```python
from build123d import *

# Parameters (mm, degrees)
SKETCH1_W           = 40
SKETCH1_H           = 10
BOSS_EXTRUDE1_DEPTH = 312.997959
SKETCH2_W           = 230.9
SKETCH2_H           = 1.2
CUT_EXTRUDE1_DEPTH  = 316.701951749
SKETCH3_R           = 1.9177
CUT_EXTRUDE2_DEPTH  = 316.701951749
CUT_EXTRUDE3_DEPTH  = 4.3
SKETCH5_R           = 2.762258299
CUT_EXTRUDE4_DEPTH  = 316.701951749
SKETCH6_W           = 3.15468
SKETCH6_H           = 6.8326
CUT_EXTRUDE5_DEPTH  = 15


with BuildPart() as part:
    # Sketch1 → Boss-Extrude1 (new body)
    with BuildSketch(Plane(origin=(0, 0, 0), x_dir=(0, 0, -1), z_dir=(1, 0, 0))):
        with Locations((20, 5)):
            Rectangle(SKETCH1_W, SKETCH1_H)
    extrude(amount=BOSS_EXTRUDE1_DEPTH)

    # Sketch2 → Cut-Extrude1 (cut, through all)
    with BuildSketch(Plane(origin=(0, 0, -40), x_dir=(-1, 0, 0), z_dir=(0, 0, -1))):
        with Locations((-156.4989795, 2.6)):
            Rectangle(SKETCH2_W, SKETCH2_H)
    extrude(amount=-CUT_EXTRUDE1_DEPTH, mode=Mode.SUBTRACT)

    # Sketch3 → Cut-Extrude2 (cut, through all)
    with BuildSketch(Plane(origin=(0, 10, 0), x_dir=(1, 0, 0), z_dir=(0, 1, 0))):
        with Locations(Location((294.997959, 25.5, 0), (0, 0, 270))):
            Circle(SKETCH3_R)
        with Locations(Location((294.997959, 14.5, 0), (0, 0, 270))):
            Circle(SKETCH3_R)
        with Locations(Location((18, 14.5, 0), (0, 0, 90))):
            Circle(SKETCH3_R)
        with Locations(Location((18, 25.5, 0), (0, 0, 90))):
            Circle(SKETCH3_R)
    extrude(amount=-CUT_EXTRUDE2_DEPTH, mode=Mode.SUBTRACT)

    # Sketch4 → Cut-Extrude3 (cut)
    with BuildSketch(Plane.XZ):
        Polygon((14.5837, -12.527598275), (14.5837, -16.472401725), (18, -18.444803449), (21.4163, -16.472401725), (21.4163, -12.527598275), (18, -10.555196551), align=None)
        Polygon((14.5837, -23.527598275), (14.5837, -27.472401725), (18, -29.444803449), (21.4163, -27.472401725), (21.4163, -23.527598275), (18, -21.555196551), align=None)
        Polygon((298.414259, -12.527598275), (294.997959, -10.555196551), (291.581659, -12.527598275), (291.581659, -16.472401725), (294.997959, -18.444803449), (298.414259, -16.472401725), align=None)
        Polygon((291.581659, -23.527598275), (291.581659, -27.472401725), (294.997959, -29.444803449), (298.414259, -27.472401725), (298.414259, -23.527598275), (294.997959, -21.555196551), align=None)
    extrude(amount=-CUT_EXTRUDE3_DEPTH, mode=Mode.SUBTRACT)

    # Sketch5 → Cut-Extrude4 (cut, through all)
    with BuildSketch(Plane.XY):
        with Locations((7, 5)):
            Circle(SKETCH5_R)
        with Locations(Location((305.997959, 5, 0), (0, 0, 180))):
            Circle(SKETCH5_R)
    extrude(amount=-CUT_EXTRUDE4_DEPTH, mode=Mode.SUBTRACT)

    # Sketch6 → Cut-Extrude5 (cut)
    with BuildSketch(Plane.ZY):
        with Locations((-31.42266, 5)):
            Rectangle(SKETCH6_W, SKETCH6_H)
        with Locations((-8.57734, 5)):
            Rectangle(SKETCH6_W, SKETCH6_H)
    extrude(amount=-CUT_EXTRUDE5_DEPTH, mode=Mode.SUBTRACT)


solid = part.part
```
Can you work these out from the model? Positions are in its coordinate system, mm. A direction names the side the tool comes from. Coordinates: 2 decimals unless noted, no trailing zeros. Loops run counter-clockwise (first coordinate to the right, second up) from the corner with the lowest first, then second, coordinate; pieces in that order, holes last. Notation, with made-up numbers: (51.25, 79) -> (78.25, 79) arc R22 cw to (78.25, 105) -> close; hole circle Ø8 at (-31, 38.5). An arc over 180 degrees is marked (long way). Put each result on its own line as item: value. Start each with the question number.
Q1. I want a section at B-B (z = -3). Write out the boundary of the cut face in (x, y).
Q2. I want a section at C-C (x = 95.5). Write out the boundary of the cut face in (y, z).
Q3. I want a section at A-A (x = 7). Write out the boundary of the cut face in (y, z).
Q4. I'm going to push a flat-ended pin straight in: P1, Ø2, axis at x = 293.5, z = -15.5, coming from the -Y side. Where does the tip first touch, or does it pass through?
Q5. For faces 4 (the face through (296.5, 4.3, -16.2)), 5 (the face through (9.1, 7.2, -29.845)), 6 (the face through (158, 2, -20)), 7 (the face through (154, 5, -40)), which set-ups out of +Z, -Z, +X, -X, +Y, -Y let a thin tool reach every point of the face, with its end or its side?
Q6. If I drill on line 1 (X direction, y = 8.4, z = -14.5); line 2 (X direction, y = 0.5, z = -25); line 3 (Y direction, x = 236, z = -22.5), over which ranges is the centre line in solid material (lowest first)? Write a range as [from, to].
Q7. Thinking about a two-plate mould opening in Y: for faces 1 (the face through (154, 10, -20)), 2 (the face through (9.1, 7.2, -7)), 3 (the face through (154, 5, 0)), which applies, pulls with the +Y half, pulls with the -Y half, needs draft (parallel to the pull), parting line crosses it, or undercut?
Taken from the geometry:
1. outline: (0, 0) -> (313, 0) -> (313, 10) -> (0, 10) -> close; hole circle Ø5.52 at (7, 5); hole (41.05, 2) -> (271.95, 2) -> (271.95, 3.2) -> (41.05, 3.2) -> close; hole circle Ø5.52 at (306, 5)
2. outline: (0, -40) -> (2, -40) -> (2, 0) -> (0, 0) -> close; (3.2, -40) -> (10, -40) -> (10, 0) -> (3.2, 0) -> close
3. outline: (0, -40) -> (2.24, -40) -> (2.24, -33) -> (1.58, -33) -> (1.58, -29.85) -> (2.24, -29.85) -> (2.24, -10.15) -> (1.58, -10.15) -> (1.58, -7) -> (2.24, -7) -> (2.24, 0) -> (0, 0) -> close; (7.76, -40) -> (10, -40) -> (10, 0) -> (7.76, 0) -> (7.76, -7) -> (8.42, -7) -> (8.42, -10.15) -> (7.76, -10.15) -> (7.76, -29.85) -> (8.42, -29.85) -> (8.42, -33) -> (7.76, -33) -> close
4. P1: stops at y = 4.3
5. face 4: -Y
5. face 5: -X
5. face 6: +Z, -Z
5. face 7: -Z, +X, -X, +Y, -Y
6. line 1: x = [0, 16.08], [19.92, 293.08], [296.92, 313]
6. line 2: x = [0, 14.58], [21.42, 291.58], [298.41, 313]
6. line 3: y = [0, 2], [3.2, 10]
7. face 1: pulls with the +Y half
7. face 2: undercut
7. face 3: needs draft
